The listing builds one solid part. Answer for the finished solid, in the listing's coordinates (mm). Coordinates: 2 decimals unless noted, no trailing zeros. Order: outer loops, then holes, each group sorted by start corner. A loop starts at its lowest first (then second) coordinate and runs counter-clockwise, first axis right, second up. Notation, with made-up numbers: (37, 78) -> (45, 78) arc R23 ccw to (45, 113) -> close; hole circle Ø9 at (52, 3). An arc over 180 degrees is marked (long way). Answer in a Markdown table with one row per item.
Autodesk Inventor part; units mm, degrees
ref_plane "YZ Plane" through (0, 0, 0) normal (1, 0, 0) x (0, 1, 0)
ref_plane "XZ Plane" through (0, 0, 0) normal (0, 1, 0) x (-1, 0, 0)
ref_plane "XY Plane" through (0, 0, 0) normal (0, 0, 1) x (1, 0, 0)
sketch "Sketch1" plane through (0, 0, 0) normal (0, 1, 0) x (-1, 0, 0)
  circle A0 centre (0, 0) radius 35.38
  dimension "d0" = 70.76
extrude "Extrusion1" add sketch "Sketch1" along normal blind 100 draft 4
shell "Shell1" thickness 0.76 removed faces 2 at (-8.491, 0, -6.3213) at (-14.5373, 100, 13.4329)
properties part number "A"
(1) Flat-ended cylindrical pins translate along their axes: pin 1 (12 mm diameter, centred on y = 20, z = -6, fed in from -X); pin 2 (3 mm diameter, centred on x = -4, y = 38, fed in from +Z); pin 3 (10 mm diameter, centred on x = 29.5, y = 60.5, fed in from +Z). Find the tip coordinate at first contact, or state that the pin passes through.
Check values:
| item | result |
|---|---|
| pin 1 | x = -37.04 |
| pin 2 | z = 38 |
| pin 3 | z = 31.15 |
(2) A cutting plane is placed at B-B, the plane z = 0. Determine the outline of the cut face in (x, y), then the cut area to 3 significant figures.
Check values:
| item | result |
|---|---|
| outline | (-42.37, 100) -> (-35.38, 0) -> (-34.62, 0) -> (-41.61, 100) -> close; (34.62, 0) -> (35.38, 0) -> (42.37, 100) -> (41.61, 100) -> close |
| area | 152 mm² |
(3) A cutting plane is placed at D-D, the plane y = 15. Determine the outline of the cut face in (x, z).
Check values:
| item | result |
|---|---|
| outline | circle Ø72.86 at (0, 0); hole circle Ø71.33 at (0, 0) |
(4) For a pull along X with two mould halves and no side action, classify faces 1 (the conical face through (8.273, 50.7, -37.256)), 2 (the flat face through (-28, 100, -31)), 3 (the conical face through (-37.13, 50.7, 11.69)) as released by +X, released by -X, zero draft, split by the parting line, or undercut.
Check values:
| item | result |
|---|---|
| face 1 | undercut |
| face 2 | zero draft |
| face 3 | split by the parting line |
(5) Find the intervals of material crossed by line 1 along Z through (x, y) = (29.5, 25); line 2 along X through (y, z) = (94, 8); line 3 along Z through (x, y) = (-27, 59), in increasing order. Write a range as from..to.
Check values:
| item | result |
|---|---|
| line 1 | -22.54..-21.27, 21.27..22.54 |
| line 2 | -41.18..-40.41, 40.41..41.18 |
| line 3 | -28.84..-27.79, 27.79..28.84 |
(6) A cutting plane is placed at A-A, the plane x = 0. Determine the outline of the cut face in (y, z), then the cut area to 3 significant figures.
Check values:
| item | result |
|---|---|
| outline | (0, -35.38) -> (100, -42.37) -> (100, -41.61) -> (0, -34.62) -> close; (0, 34.62) -> (100, 41.61) -> (100, 42.37) -> (0, 35.38) -> close |
| area | 152 mm² |
(7) A cutting plane is placed at C-C, the plane y = 42. Determine the outline of the cut face in (x, z).
Check values:
| item | result |
|---|---|
| outline | circle Ø76.63 at (0, 0); hole circle Ø75.11 at (0, 0) |
